Part print with two shaded views. Sizes in mm from the minimum x, y, z corner. Give positions to 0.01 mm unless a question says otherwise; leave off trailing zeros. Write each loop counter-clockwise with the first axis right and the second up, starting at its lowest first coordinate (ties: lowest second). Pieces come first, ordered by that corner, then holes. Notation, with made-up numbers: (-12.5, -17) - (18.5, -17) arc R8 ccw to (18.5, -3) - close; hole circle Ø3 at (-33, 17). An arc over 180 degrees is marked (long way). One line per item, written item: value. Start each with the question number.
(1) Probe L1, parallel to X at y = 1.35, z = 12.5; L2, parallel to X at y = 1.65, z = 19; L3, parallel to Z at x = 7.75, y = 1.5. List the from-to ranges inside material, lowest first.
(2) Cut at A-A, the plane z = 12.75. List the corners of the cut face in (x, y).
(3) Cut at B-B, the plane z = 19.75. List the corners of the cut face in (x, y), and give its area (3 significant figures).
(4) Cut at C-C, the plane y = 0.7. List the corners of the cut face in (x, z).
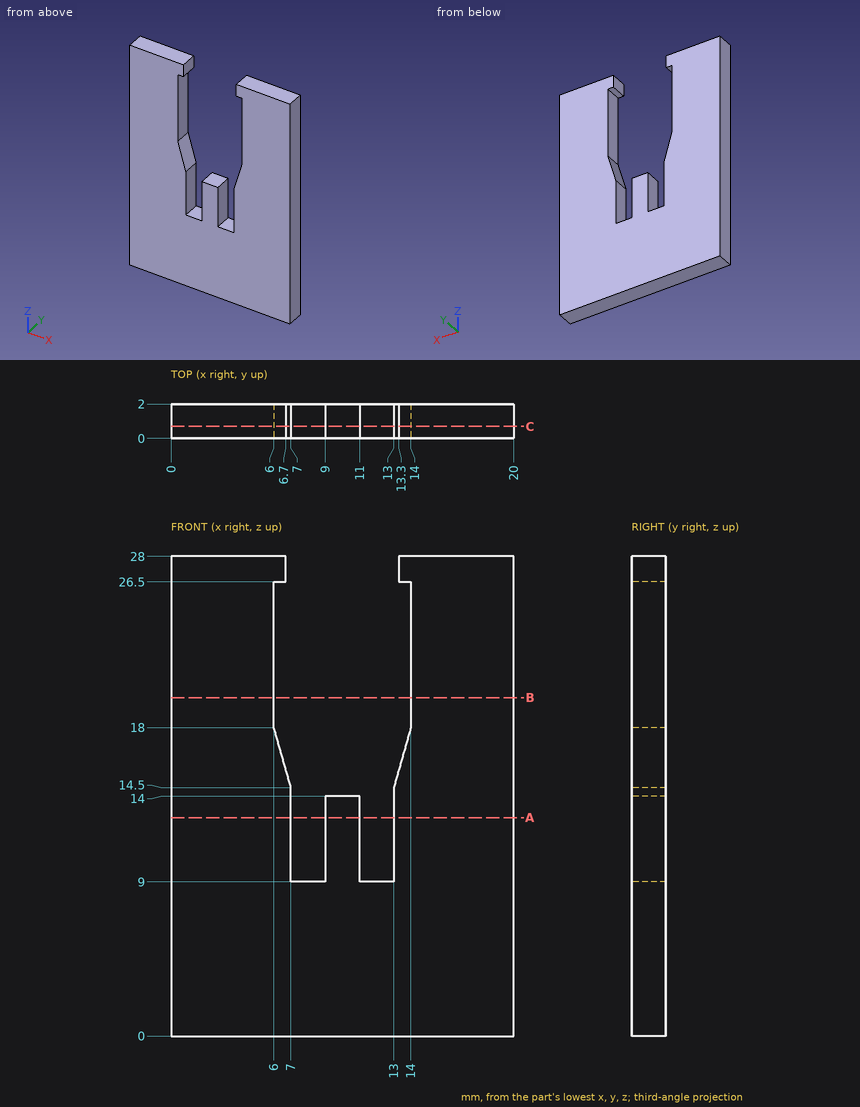
Answers follow:
1. L1: x = 0 to 7, 9 to 11, 13 to 20
1. L2: x = 0 to 6, 14 to 20
1. L3: z = 0 to 9
2. outline: (0, 0) - (7, 0) - (7, 2) - (0, 2) - close; (9, 0) - (11, 0) - (11, 2) - (9, 2) - close; (13, 0) - (20, 0) - (20, 2) - (13, 2) - close
3. outline: (0, 0) - (6, 0) - (6, 2) - (0, 2) - close; (14, 0) - (20, 0) - (20, 2) - (14, 2) - close
3. area: 24.0 mm²
4. outline: (0, 0) - (20, 0) - (20, 28) - (13.3, 28) - (13.3, 26.5) - (14, 26.5) - (14, 18) - (13, 14.5) - (13, 9) - (11, 9) - (11, 14) - (9, 14) - (9, 9) - (7, 9) - (7, 14.5) - (6, 18) - (6, 26.5) - (6.7, 26.5) - (6.7, 28) - (0, 28) - close
